Design review of the part shown in the three views and the two pictorial views. Dimensions are in mm from the part's minimum x, y and z. Give positions to 0.01 mm unless a question says otherwise; leave off trailing zeros. Order: outer loops, then holes, each group sorted by start corner. A loop starts at its lowest first (then second) coordinate and runs counter-clockwise, first axis right, second up.
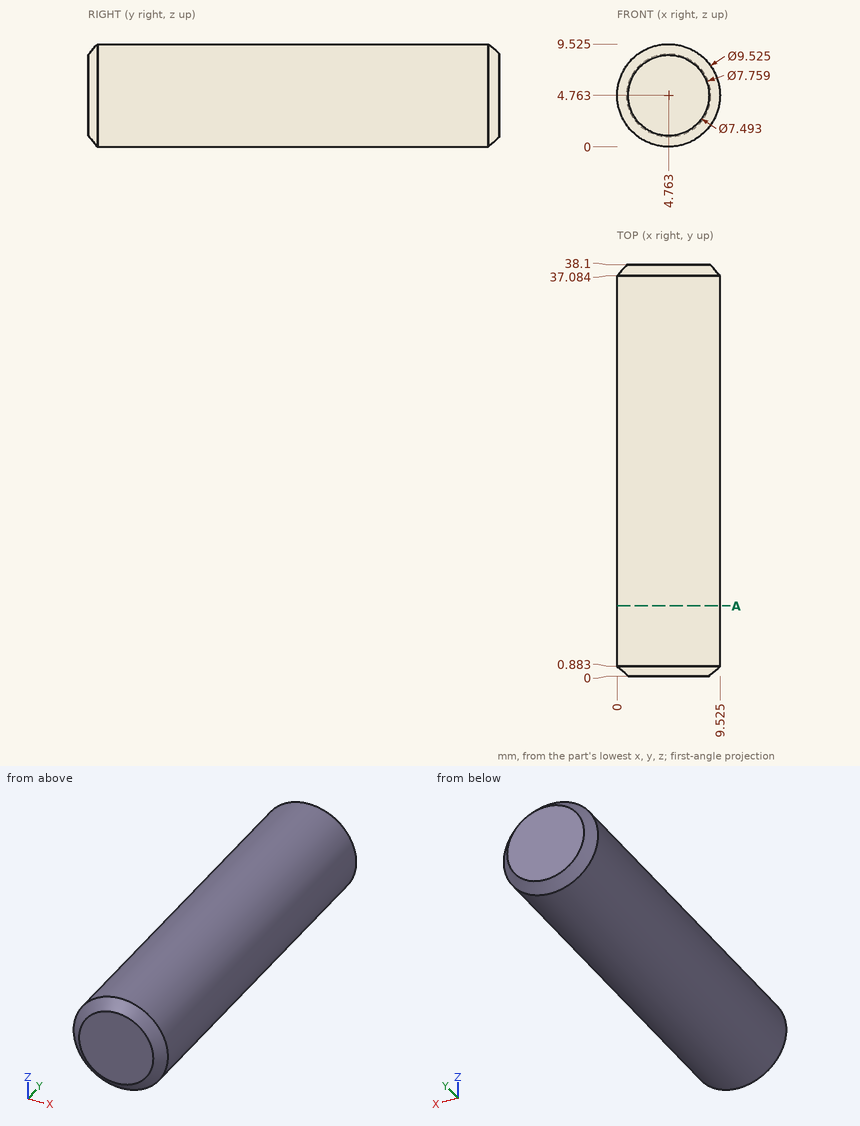
1) We need section A-A on y = 6.5. Give the boundary of the cut face in (x, z) (1 decimal).
Answer sheet:
outline: circle Ø9.5 at (4.8, 4.8)
2) To check wall thickness, follow line 1 (Y direction, x = 2.5, z = 7.75); line 2 (Z direction, x = 5.25, y = 30.5) (1 decimal); line 3 (X direction, y = 2.5, z = 9) (1 decimal). State the ranges of each line that lie inside material, in increasing order.
Answer sheet:
line 1: y = 0 to 38.1
line 2: z = 0 to 9.5
line 3: x = 2.6 to 6.9
3) Clearance check with flat-ended pins moving along their axes: pin 1 (3 mm diameter, centred on x = 1.5, y = 4.5, fed in from +Z); pin 2 (1.5 mm diameter, centred on x = 2, y = 32, fed in from -Z) (1 decimal). State where each tip first meets the part, or that it passes through.
Answer sheet:
pin 1: stops at z = 9.19
pin 2: stops at z = 0.4
